Could you check a few things on this model? Use its own coordinates, in mm. A direction names the side the tool comes from. Coordinates: 2 decimals unless noted, no trailing zeros. Order: outer loops, then holes, each group sorted by start corner. A loop starts at its lowest first (then second) coordinate and runs counter-clockwise, first axis right, second up. Notation, with made-up numbers: (47.5, 7.5) -> (82.5, 7.5) arc R4 ccw to (82.5, 13.5) -> close; hole circle Ø7 at (-26, 48.25). An arc over 180 degrees is marked (long way). Put each result on its own line as item: value. Start each with the question number.
Q1. If we section it at C-C (z = -39.5): Please give me the cut outline in (x, y).
Q2. If we section it at B-B (y = 28): Please give me the cut outline in (x, z), and give its area (3 significant figures).
Q3. We'd pull the mould along X, two halves only. Please class faces 5 (the face through (-149.997, 17.748, -1.02)), 6 (the face through (-96, 3, -60)), 7 (the face through (-121, 1, -28)): +X half, -X half, draft (parallel to the pull), parting line (faces both ways), or undercut.
Q4. Will these pins go through, and if not, where does the flat tip stop? pin 1 (1 mm diameter, centred on y = 28, z = -48.5, fed in from +X); pin 2 (1.5 mm diameter, centred on x = -42, y = 4.5, fed in from -Z); pin 3 (3.5 mm diameter, centred on y = 1, z = -21.5, fed in from +X).
Q5. If we section it at D-D (x = -128.5): Please give me the cut outline in (y, z).
Q6. If we section it at A-A (x = -57): Please give me the cut outline in (y, z), and give its area (3 significant figures).
Q7. For faces 1 (the face through (-40, 4, 50)), 2 (the face through (-40, 4, -50)), 3 (the face through (-131, 1, -6)), 4 (the face through (-96, 1, 50)), which set-ups out of +Z, -Z, +X, -X, +Y, -Y let a thin tool reach every point of the face, with its end or its side?
Q8. Please list where these lines run through material, in increasing order: line 1 along Y through (x, z) = (-74.5, 51); line 2 along Y through (x, z) = (-105.5, -5); line 3 along X through (y, z) = (34, -2).
from build123d import *

# Parameters (mm, degrees)
BOSS_EXTRUDE1_DEPTH = 6
BOSS_EXTRUDE2_DEPTH = 30
SKETCH3_W           = 20
SKETCH3_H           = 100
CUT_EXTRUDE1_DEPTH  = 3
SHELL1_START        = 2
SHELL1_DEPTH        = 32
SHELL1_START_2      = 5
SHELL1_2_OUTLINE_W  = 2
SHELL1_2_OUTLINE_H  = 96
SHELL1_2_DEPTH      = 29
BOSS_EXTRUDE3_DEPTH = 6
CUT_EXTRUDE2_START  = -2
CUT_EXTRUDE2_DEPTH  = 2
SKETCH8_W           = 21
SKETCH8_H           = 44
CUT_EXTRUDE3_DEPTH  = 3
SKETCH9_W           = 90
SKETCH9_H           = 30
CUT_EXTRUDE4_DEPTH  = 196.437969699


# Read off the part's stored shape, not the designer's step: Shell1
with BuildPart() as part:
    # Sketch1 → Boss-Extrude1 (new body)
    with BuildSketch(Plane(origin=(0, 0, 0), x_dir=(1, 0, 0), z_dir=(0, 1, 0))):
        with BuildLine():
            Line((-50, 50), (-141.421356237, 50))
            ThreePointArc((-141.421356237, 50), (-150, 0), (-141.421356237, -50))
            Line((-141.421356237, -50), (-50, -50))
            Line((-50, -50), (-50, 0))
            Line((-50, 0), (-50, 50))
        make_face()
        with BuildLine():
            Line((-50, -50), (-141.421356237, -50))
            ThreePointArc((-141.421356237, -50), (-137.407538074, -60.159525267), (-132.664991614, -70))
            Line((-132.664991614, -70), (-50, -70))
            Line((-50, -70), (-50, -50))
        make_face()
        Polygon((-30, 50), (-50, 50), (-50, 0), (-50, -50), (-30, -50), (-30, 0), align=None)
        with BuildLine():
            Line((-50, 70), (-132.664991614, 70))
            ThreePointArc((-132.664991614, 70), (-137.407538074, 60.159525267), (-141.421356237, 50))
            Line((-141.421356237, 50), (-50, 50))
            Line((-50, 50), (-50, 70))
        make_face()
    extrude(amount=BOSS_EXTRUDE1_DEPTH)

    # Sketch2 → Boss-Extrude2 (add)
    with BuildSketch(Plane(origin=(0, 6, 0), x_dir=(-1, 0, 0), z_dir=(0, 1, 0))):
        with BuildLine():
            Line((50, 50), (50, -50))
            Line((50, -50), (141.421356237, -50))
            ThreePointArc((141.421356237, -50), (150, 0), (141.421356237, 50))
            Line((141.421356237, 50), (50, 50))
        make_face()
    extrude(amount=BOSS_EXTRUDE2_DEPTH)

    # Sketch3 → Cut-Extrude1 (cut)
    with BuildSketch(Plane.XZ):
        with BuildLine():
            Line((-50, -70), (-50, -50))
            Line((-50, -50), (-141.421356237, -50))
            ThreePointArc((-141.421356237, -50), (-137.407538074, -60.159525267), (-132.664991614, -70))
            Line((-132.664991614, -70), (-50, -70))
        make_face()
        with Locations((-40, 0)):
            Rectangle(SKETCH3_W, SKETCH3_H)
        with BuildLine():
            Line((-141.421356237, 50), (-50, 50))
            Line((-50, 50), (-50, 70))
            Line((-50, 70), (-132.664991614, 70))
            ThreePointArc((-132.664991614, 70), (-137.407538074, 60.159525267), (-141.421356237, 50))
        make_face()
    extrude(amount=-CUT_EXTRUDE1_DEPTH, mode=Mode.SUBTRACT)

    # Shell1 outline → Shell1 (cut)
    with BuildSketch(Plane(origin=(0, 0, 0), x_dir=(1, 0, 0), z_dir=(0, 1, 0)).offset(SHELL1_START)):
        with BuildLine():
            Line((-140, -48), (-52, -48))
            Line((-52, -48), (-52, 48))
            Line((-52, 48), (-140, 48))
            ThreePointArc((-140, 48), (-148, 0), (-140, -48))
        make_face()
    extrude(amount=SHELL1_DEPTH, mode=Mode.SUBTRACT)

    # Shell1 2 outline → Shell1 2 (cut)
    with BuildSketch(Plane(origin=(0, 0, 0), x_dir=(1, 0, 0), z_dir=(0, 1, 0)).offset(SHELL1_START_2)):
        with Locations((-51, 0)):
            Rectangle(SHELL1_2_OUTLINE_W, SHELL1_2_OUTLINE_H)
    extrude(amount=SHELL1_2_DEPTH, mode=Mode.SUBTRACT)

    # Sketch6 → Boss-Extrude3 (add)
    with BuildSketch(Plane.XZ):
        with BuildLine():
            Line((-141.421356237, 50), (-50, 50))
            Line((-50, 50), (-50, -50))
            Line((-50, -50), (-141.421356237, -50))
            ThreePointArc((-141.421356237, -50), (-150, 0), (-141.421356237, 50))
        make_face()
    extrude(amount=-BOSS_EXTRUDE3_DEPTH)

    # Sketch7 → Cut-Extrude2 (cut)
    with BuildSketch(Plane(origin=(0, 36, 0), x_dir=(-1, 0, 0), z_dir=(0, 1, 0)).offset(CUT_EXTRUDE2_START)):
        with BuildLine():
            Line((50, -48), (140, -48))
            ThreePointArc((140, -48), (148, 0), (140, 48))
            Line((140, 48), (50, 48))
            Line((50, 48), (50, -48))
        make_face()
    extrude(amount=CUT_EXTRUDE2_DEPTH, mode=Mode.SUBTRACT)

    # Sketch8 → Cut-Extrude3 (cut)
    with BuildSketch(Plane.XZ):
        with Locations((-120.5, -6)):
            Rectangle(SKETCH8_W, SKETCH8_H)
    extrude(amount=-CUT_EXTRUDE3_DEPTH, mode=Mode.SUBTRACT)

    # Sketch9 → Cut-Extrude4 (cut, through all)
    with BuildSketch(Plane.XY.offset(50)):
        with Locations((-95, 21)):
            Rectangle(SKETCH9_W, SKETCH9_H)
    extrude(amount=-CUT_EXTRUDE4_DEPTH, mode=Mode.SUBTRACT)


solid = part.part
The answers:
1. outline: (-144.71, 0) -> (-50, 0) -> (-50, 3) -> (-30, 3) -> (-30, 6) -> (-142.63, 6) -> (-142.63, 36) -> (-144.71, 36) -> close
2. outline: (-141.42, -50) -> (-140, -50) -> (-140, -48) arc R148 cw to (-140, 48) -> (-140, 50) -> (-141.42, 50) arc R150 ccw to start
2. area: 203 mm^2
3. face 5: -X half
3. face 6: draft
3. face 7: undercut
4. pin 1: x = -140
4. pin 2: z = -50
4. pin 3: x = -50
5. outline: (0, -50) -> (3, -50) -> (3, -70) -> (6, -70) -> (6, 70) -> (3, 70) -> (3, 50) -> (0, 50) -> (0, 16) -> (3, 16) -> (3, -28) -> (0, -28) -> close
6. outline: (0, -50) -> (3, -50) -> (3, -70) -> (6, -70) -> (6, 70) -> (3, 70) -> (3, 50) -> (0, 50) -> close
6. area: 720 mm^2
7. face 1: +Z, +X, +Y, -Y
7. face 2: -Z, +X, +Y, -Y
7. face 3: -Y
7. face 4: +Z, +X, -X, -Y
8. line 1: 3 to 6
8. line 2: 0 to 6
8. line 3: -149.99 to -147.99
